Geometry check sheet. Reference: the model listing, model coordinates, mm. Round coordinates to 2 decimals unless told otherwise and drop trailing zeros. Write each loop counter-clockwise with the first axis right and the second up, starting at its lowest first coordinate (ties: lowest second). Pieces come first, ordered by that corner, then holes. Notation, with made-up numbers: M 24.25,63 L 75.25,63 A31 ccw 75.25,100 Z; hole C -22,60 d9. An arc over 180 degrees is marked long. One line per item, written item: value. Start each with the question number.
1. Scan lines: probe 1 along X at (y, z) = (2, -15.5); probe 2 along Z at (x, y) = (35, 1.3); probe 3 along Z at (x, y) = (-10, 2). Record each from-to range of solid material in increasing order. Write a range as [from, to].
2. Section check B-B (y = 1.4). Count the separate pieces of the cut face and the enclosed holes in it, and give its area (3 significant figures).
3. Section check C-C (x = 14). Record the boundary of the cut face in (y, z), and give its area (3 significant figures).
4. Depth check by flat-ended pin: P1, Ø0.9, axis at y = 1.5, z = 19, coming from the -X side; P2, Ø1, axis at x = -17.5, y = 1.5, coming from the +Z side; P3, Ø1.5, axis at x = 44.5, y = 2, coming from the -Z side; P4, Ø12, axis at x = -4, z = -2.5, coming from the -Y side. Enter the tip coordinate at first touch or a pass-through.
5. Section check A-A (x = -30). Record the boundary of the cut face in (y, z), and give its area (3 significant figures).
from build123d import *

# Parameters (mm, degrees)
BOSS_EXTRUDE1_DEPTH = 3
SKETCH2_W           = 14
SKETCH2_H           = 12.5
CUT_EXTRUDE1_DEPTH  = 10


with BuildPart() as part:
    # Sketch1 → Boss-Extrude1 (new body)
    with BuildSketch(Plane(origin=(0, 0, 0), x_dir=(1, 0, 0), z_dir=(0, 1, 0))):
        Polygon((-42.760092083, 15.020184167), (-42.760092083, 4.645184167), (-45.760092083, 4.645184167), (-45.760092083, -9.604815833), (-42.760092083, -9.604815833), (-42.760092083, -16.979815833), (-35.885092083, -16.979815833), (-35.885092083, -19.979815833), (-21.635092083, -19.979815833), (-21.635092083, -16.979815833), (-7.385092083, -16.979815833), (-7.385092083, -19.979815833), (6.864907917, -19.979815833), (6.864907917, -16.979815833), (21.114907917, -16.979815833), (21.114907917, -19.979815833), (35.364907917, -19.979815833), (35.364907917, -16.979815833), (42.239907917, -16.979815833), (42.239907917, -9.604815833), (45.239907917, -9.604815833), (45.239907917, 4.645184167), (42.239907917, 4.645184167), (42.239907917, 15.020184167), (35.364907917, 15.020184167), (35.364907917, 18.020184167), (21.114907917, 18.020184167), (21.114907917, 15.020184167), (6.864907917, 15.020184167), (6.864907917, 18.020184167), (-7.385092083, 18.020184167), (-7.385092083, 15.020184167), (-21.635092083, 15.020184167), (-21.635092083, 18.020184167), (-35.885092083, 18.020184167), (-35.885092083, 15.020184167), align=None)
    extrude(amount=BOSS_EXTRUDE1_DEPTH)

    # Sketch2 → Cut-Extrude1 (cut)
    with BuildSketch(Plane(origin=(0, 3, 0), x_dir=(1, 0, 0), z_dir=(0, 1, 0))):
        with Locations((30.239907917, 5.770184167)):
            Rectangle(SKETCH2_W, SKETCH2_H)
        with BuildLine():
            Line((-37, 12.998362663), (0, 12.998362663))
            ThreePointArc((0, 12.998362663), (3.5, 9.498362663), (0, 5.998362663))
            Line((0, 5.998362663), (-37, 5.998362663))
            ThreePointArc((-37, 5.998362663), (-40.5, 9.498362663), (-37, 12.998362663))
        make_face()
    extrude(amount=-CUT_EXTRUDE1_DEPTH, mode=Mode.SUBTRACT)


solid = part.part
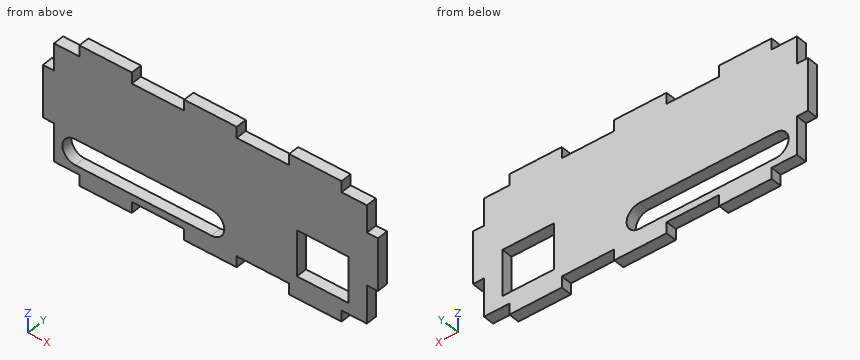
Result sheet:
1. probe 1: x = [-35.89, -21.64], [-7.39, 6.86], [21.11, 35.36]
1. probe 2: z = [-18.02, -12.02], [0.48, 19.98]
1. probe 3: z = [-15.02, -13], [-6, 16.98]
2. separate pieces: 1
2. enclosed holes: 2
2. area: 2,590 mm2
3. outline: M 0,-15.02 L 3,-15.02 L 3,16.98 L 0,16.98 Z
3. area: 96.0 mm2
4. P1: stops at x = -35.89
4. P2: stops at z = 16.98
4. P3: stops at z = -4.65
4. P4: stops at y = 0
5. outline: M 0,-18.02 L 3,-18.02 L 3,-13 L 0,-13 Z; M 0,-6 L 3,-6 L 3,19.98 L 0,19.98 Z
5. area: 93.0 mm2
